The listing builds one solid part. Answer for the finished solid, in the listing's coordinates (mm). A direction names the side the tool comes from. Coordinates: 2 decimals unless noted, no trailing zeros. Write each loop counter-clockwise with the first axis right and the second up, starting at its lowest first coordinate (ties: lowest second). Pieces come first, ordered by that corner, then holes.
(1) Given P1, Ø3, axis at x = -80, y = 30, coming from the -Z side; P2, Ø0.6, axis at x = -10.5, z = -1.5, coming from the +Y side; P3, Ø0.6, axis at y = -21, z = -1, coming from the +X side, each flat-ended and moving along its own axis, determine where each tip first touches the part or whether it passes through.
(2) The part is cut by section A-A on y = 21. Determine the outline of the cut face in (x, z), plus the area to 3 significant figures.
(3) Straight lines are drawn through the part: line 1 (Y direction, x = -80, z = 1.6); line 2 (X direction, y = 15.5, z = 3.5); line 3 (Y direction, x = -13, z = 2). For each, find the intervals that lie inside material, in ascending order.
(4) The part is cut by section D-D on y = 0. Determine the outline of the cut face in (x, z), plus the area to 3 significant figures.
(5) Which of the six approach directions +Z, -Z, +X, -X, +Y, -Y give full straight-line access (tool end or side, diameter ignored) to faces 1 (the cylindrical face through (83, -34, 3)), 2 (the flat face through (-16.5, 15, 2))?
(6) For a pull along Y with two mould halves and no side action, classify faces 3 (the cylindrical face through (-84, -33, 3)), 4 (the flat face through (-18, -15, 1)), 5 (the flat face through (-1, 0, 0)), 6 (the flat face through (0, -20.04, 1)) as +Y half, -Y half, draft (parallel to the pull), parting line (faces both ways), or undercut.
(7) The part is cut by section B-B on z = 3.25. Determine the outline of the cut face in (x, y).
(8) The part is cut by section C-C on x = -23.5. Determine the outline of the cut face in (y, z), plus the area to 3 significant figures.
from build123d import *

# Parameters (mm, degrees)
SKETCH1_W           = 170
SKETCH1_H           = 70
BOSS_EXTRUDE1_DEPTH = 5
FILLET2_R           = 5
SKETCH3_R           = 1.4
CUT_EXTRUDE1_DEPTH  = 5
SKETCH5_R           = 1.4
CUT_EXTRUDE2_DEPTH  = 5
CUT_EXTRUDE5_DEPTH  = 5
CUT_EXTRUDE7_DEPTH  = 5
BOSS_EXTRUDE2_DEPTH = 10
CUT_EXTRUDE8_DEPTH  = 10
SKETCH10_W          = 3
SKETCH10_H          = 26
CUT_EXTRUDE9_DEPTH  = 57
FILLET3_R           = 2.5


with BuildPart() as part:
    # Sketch1 → Boss-Extrude1 (new body)
    with BuildSketch(Plane.XY):
        Rectangle(SKETCH1_W, SKETCH1_H)
    extrude(amount=BOSS_EXTRUDE1_DEPTH)

    # Fillet2
    fillet2_edges = [part.edges().sort_by_distance(p)[0] for p in [
        (85, -35, 2.5),
        (-85, -35, 2.5),
        (-85, 35, 2.5),
        (85, 35, 2.5),
    ]]
    fillet(fillet2_edges, radius=FILLET2_R)

    # Sketch3 → Cut-Extrude1 (cut)
    with BuildSketch(Plane.XY):
        with Locations((-80, 30)):
            Circle(SKETCH3_R)
    extrude(amount=CUT_EXTRUDE1_DEPTH, mode=Mode.SUBTRACT)

    # Sketch5 → Cut-Extrude2 (cut)
    with BuildSketch(Plane.XY.offset(5)):
        with Locations((-80, -30)):
            Circle(SKETCH5_R)
        with Locations((80, 30)):
            Circle(SKETCH5_R)
        with Locations((80, -30)):
            Circle(SKETCH5_R)
    extrude(amount=-CUT_EXTRUDE2_DEPTH, mode=Mode.SUBTRACT)

    # Sketch6 → Cut-Extrude5 (cut)
    with BuildSketch(Plane.XY):
        Polygon((0, 7.806871993), (16.5, 7.806871993), (16.5, 22.806871993), (-16.5, 22.806871993), (-16.5, 7.806871993), align=None)
    extrude(amount=CUT_EXTRUDE5_DEPTH, mode=Mode.SUBTRACT)

    # Sketch7 → Cut-Extrude7 (cut)
    with BuildSketch(Plane.XY):
        Polygon((-65, 15.306871993), (-65, 22.506871993), (-57, 22.506871993), (-57, 15.306871993), (-57, 8.106871993), (-65, 8.106871993), align=None)
    extrude(amount=CUT_EXTRUDE7_DEPTH, mode=Mode.SUBTRACT)

    # Sketch8 → Boss-Extrude2 (add)
    with BuildSketch(Plane.XY.offset(5)):
        Polygon((0, -2), (28.5, -2), (28.5, -14.153073617), (28.5, -28), (-28.5, -28), (-28.5, -14.153073617), (-28.5, -2), align=None)
    extrude(amount=-BOSS_EXTRUDE2_DEPTH)

    # Sketch9 → Cut-Extrude8 (cut)
    with BuildSketch(Plane(origin=(0, 0, -5), x_dir=(-1, 0, 0), z_dir=(0, 0, -1))):
        Polygon((18, -20.04), (-18, -20.04), (-18, -15), (-18, -9.96), (18, -9.96), (18, -15), align=None)
    extrude(amount=-CUT_EXTRUDE8_DEPTH, mode=Mode.SUBTRACT)

    # Sketch10 → Cut-Extrude9 (cut)
    with BuildSketch(Plane(origin=(28.5, 0, 0), x_dir=(0, 0, -1), z_dir=(1, 0, 0))):
        with Locations((3.5, -15)):
            Rectangle(SKETCH10_W, SKETCH10_H)
    extrude(amount=-CUT_EXTRUDE9_DEPTH, mode=Mode.SUBTRACT)

    # Fillet3
    fillet3_edges = [part.edges().sort_by_distance(p)[0] for p in [
        (18, -9.96, 1.5),
        (-18, -9.96, 1.5),
        (-18, -20.04, 1.5),
        (18, -20.04, 1.5),
    ]]
    fillet(fillet3_edges, radius=FILLET3_R)


solid = part.part
Model answer:
1. P1: stops at z = 0
1. P2: stops at y = -2
1. P3: stops at x = 28.5
2. outline: (-85, 0) - (-65, 0) - (-65, 5) - (-85, 5) - close; (-57, 0) - (-16.5, 0) - (-16.5, 5) - (-57, 5) - close; (16.5, 0) - (85, 0) - (85, 5) - (16.5, 5) - close
2. area: 645 mm2
3. line 1: y = -35 to -31.4, -28.6 to 28.6, 31.4 to 35
3. line 2: x = -85 to -65, -57 to -16.5, 16.5 to 85
3. line 3: y = -35 to -20.04, -9.96 to 7.81, 22.81 to 35
4. outline: (-85, 0) - (85, 0) - (85, 5) - (-85, 5) - close
4. area: 850 mm2
5. face 1: +Z, -Z, +X, -Y
5. face 2: +Z, -Z
6. face 3: -Y half
6. face 4: undercut
6. face 5: draft
6. face 6: undercut
7. outline: (-85, -30) arc R5 ccw to (-80, -35) - (80, -35) arc R5 ccw to (85, -30) - (85, 30) arc R5 ccw to (80, 35) - (-80, 35) arc R5 ccw to (-85, 30) - close; hole circle Ø2.8 at (-80, -30); hole circle Ø2.8 at (-80, 30); hole (-65, 8.11) - (-57, 8.11) - (-57, 22.51) - (-65, 22.51) - close; hole (-18, -17.54) arc R2.5 ccw to (-15.5, -20.04) - (15.5, -20.04) arc R2.5 ccw to (18, -17.54) - (18, -12.46) arc R2.5 ccw to (15.5, -9.96) - (-15.5, -9.96) arc R2.5 ccw to (-18, -12.46) - close; hole (-16.5, 7.81) - (16.5, 7.81) - (16.5, 22.81) - (-16.5, 22.81) - close; hole circle Ø2.8 at (80, -30); hole circle Ø2.8 at (80, 30)
8. outline: (-35, 0) - (-28, 0) - (-28, -2) - (-2, -2) - (-2, 0) - (35, 0) - (35, 5) - (-35, 5) - close
8. area: 402 mm2
